Geometry: final body of the model. Coordinates: model frame, mm. Give positions to 0.01 mm unless a question says otherwise; leave off trailing zeros. Loops run counter-clockwise (first coordinate to the right, second up) from the corner with the lowest first, then second, coordinate; pieces in that order, holes last. Notation, with made-up numbers: (8, 25) - (41, 25) arc R21 cw to (41, 39) - close; hole circle Ø3 at (65, -8.5). An arc over 180 degrees is marked (long way). Use one line per item in the form item = value.
```python
from build123d import *

# Parameters (mm, degrees)
SKETCH_1_W      = 50
SKETCH_1_H      = 150
SKETCH_1_R      = 1.6
EXTRUDE_1_DEPTH = 4


with BuildPart() as part:
    # 草图1 → 凸台-拉伸1 (new body)
    with BuildSketch(Plane(origin=(0, 0, 0), x_dir=(1, 0, 0), z_dir=(0, 1, 0))):
        Rectangle(SKETCH_1_W, SKETCH_1_H)
        with Locations((-15, 63)):
            Circle(SKETCH_1_R, mode=Mode.SUBTRACT)
        with Locations((15, 63)):
            Circle(SKETCH_1_R, mode=Mode.SUBTRACT)
        with Locations((0, -67)):
            Circle(SKETCH_1_R, mode=Mode.SUBTRACT)
    extrude(amount=EXTRUDE_1_DEPTH)


solid = part.part
```
(1) Material intervals for L1, parallel to X at y = 1.8, z = -63; L2, parallel to Z at x = -15, y = 2.35; L3, parallel to X at y = 2.3, z = 67, sorted ascending. Write a range as from..to.
Solution:
L1 = -25..-16.6, -13.4..13.4, 16.6..25
L2 = -75..-64.6, -61.4..75
L3 = -25..-1.6, 1.6..25
(2) Pull-direction query (Z, two-part tool) for faces 1 (the face through (0, 2, -75)), 2 (the face through (0, 4, -1)), 3 (the face through (-15.208, 1.972, -64.586)); classes: released by +Z, released by -Z, zero draft, split by the parting line, or undercut.
Solution:
face_1 = released by -Z
face_2 = zero draft
face_3 = undercut
(3) Cut plane B-B (z = 67). Return the cut outline in (x, y), plus the area to 3 significant figures.
Solution:
outline = (-25, 0) - (-1.6, 0) - (-1.6, 4) - (-25, 4) - close; (1.6, 0) - (25, 0) - (25, 4) - (1.6, 4) - close
area = 187 mm2
(4) Pin query (flat end, axial travel): P1, Ø2.5, axis at x = 0, z = 67, coming from the +Y side. Return the tip coordinate at first contact, or that it passes through.
Solution:
P1 = through
(5) Cut plane A-A (x = 15). Return the cut outline in (y, z).
Solution:
outline = (0, -75) - (4, -75) - (4, -64.6) - (0, -64.6) - close; (0, -61.4) - (4, -61.4) - (4, 75) - (0, 75) - close
